CAD build for the part. Positions are in the model's coordinates, mm. A direction names the side the tool comes from. Round coordinates to 2 decimals unless told otherwise and drop trailing zeros. Loops run counter-clockwise (first coordinate to the right, second up) from the corner with the lowest first, then second, coordinate; pieces in that order, holes last. Notation, with made-up numbers: (-20.75, 62.25) - (20.25, 62.25) arc R28 ccw to (20.25, 88.25) - close; hole circle Ø6 at (-24, 36). An arc over 180 degrees is marked (long way). Use one line per item in the form item = value.
from build123d import *

# Parameters (mm, degrees)
SKETCH3_W           = 95
SKETCH3_H           = 50
SKETCH3_RX          = 2.5
SKETCH3_RY          = 2.5
SKETCH3_RX_2        = 6
SKETCH3_RY_2        = 6
SKETCH3_W_2         = 26
SKETCH3_H_2         = 17
SKETCH3_W_3         = 27
SKETCH3_H_3         = 13
SKETCH3_W_4         = 9
SKETCH3_H_4         = 16
BOSS_EXTRUDE2_DEPTH = 4


with BuildPart() as part:
    # Sketch3 → Boss-Extrude2 (new body)
    with BuildSketch(Plane.XY):
        with Locations((-63.7985, -48.7036)):
            Rectangle(SKETCH3_W, SKETCH3_H)
        with Locations(Location((-36.0722, -48.7036), (0, 0, 90))):
            Ellipse(SKETCH3_RX, SKETCH3_RY, mode=Mode.SUBTRACT)
        with Locations(Location((-100.8596, -38.7221), (0, 0, 180))):
            Ellipse(SKETCH3_RX_2, SKETCH3_RY_2, mode=Mode.SUBTRACT)
        with Locations((-74.0985, -40.2036)):
            Rectangle(SKETCH3_W_2, SKETCH3_H_2, mode=Mode.SUBTRACT)
        with Locations((-74.0985, -62.7036)):
            Rectangle(SKETCH3_W_3, SKETCH3_H_3, mode=Mode.SUBTRACT)
        with Locations((-100.8596, -58.7221)):
            Rectangle(SKETCH3_W_4, SKETCH3_H_4, mode=Mode.SUBTRACT)
    extrude(amount=BOSS_EXTRUDE2_DEPTH)


solid = part.part
1) Flat gauge pin, fed straight in: pin 1 (5 mm diameter, centred on x = -83, y = -58.5, fed in from +Z). Where does the tip first touch, or does it go through?
Report:
pin_1 = 4
2) Slice it at B-B (y = -64.5). Write the cut outline in (x, z), plus the area to 3 significant figures.
Report:
outline = (-111.3, 0) - (-105.36, 0) - (-105.36, 4) - (-111.3, 4) - close; (-96.36, 0) - (-87.6, 0) - (-87.6, 4) - (-96.36, 4) - close; (-60.6, 0) - (-16.3, 0) - (-16.3, 4) - (-60.6, 4) - close
area = 236 mm^2
3) Slice it at C-C (z = 3.05). State how many separate pieces and enclosed holes the cut face has, plus the area to 3 significant figures.
Report:
separate_pieces = 1
enclosed_holes = 5
area = 3,680 mm^2
4) Drill centre lines: probe 1 along Y at (x, z) = (-63.5, 1.5); probe 2 along X at (y, z) = (-66, 2.4); probe 3 along X at (y, z) = (-45.5, 2.15). Where is each one in solid material? Low to high.
Report:
probe_1 = -73.7 to -69.2, -56.2 to -48.7, -31.7 to -23.7
probe_2 = -111.3 to -105.36, -96.36 to -87.6, -60.6 to -16.3
probe_3 = -111.3 to -87.1, -61.1 to -16.3
5) Slice it at A-A (x = -71.5). Write the cut outline in (y, z), plus the area to 3 significant figures.
Report:
outline = (-73.7, 0) - (-69.2, 0) - (-69.2, 4) - (-73.7, 4) - close; (-56.2, 0) - (-48.7, 0) - (-48.7, 4) - (-56.2, 4) - close; (-31.7, 0) - (-23.7, 0) - (-23.7, 4) - (-31.7, 4) - close
area = 80.0 mm^2
6) Two-plate mould, pull along X, no slides. Class faces 3 (the flat face through (-64, -54, 0)), 4 (the flat face through (-16.298, -49, 2)), 5 (the flat face through (-101, -50.722, 2)), 6 (the flat face through (-74, -69.204, 2)): +X half, -X half, draft (parallel to the pull), parting line (faces both ways), or undercut.
Report:
face_3 = draft
face_4 = +X half
face_5 = undercut
face_6 = undercut
7) Tool access for faces 1 (the flat face through (-64, -54, 4)), 2 (the flat face through (-96.36, -59, 2)): list every direction of +Z, -Z, +X, -X, +Y, -Y with a clear straight run to the whole face (end or side of a thin tool).
Report:
face_1 = +Z, +X, -X, +Y, -Y
face_2 = +Z, -Z
